from build123d import *

# Parameters (mm, degrees)
F0_R     = 1.905
F1_DEPTH = 2.032
F2_DEPTH = 2.54
F3_R     = 1.016


with BuildPart() as f1:
    # F0 (on Top) → F1 (new body)
    with BuildSketch(Plane.XY):
        with BuildLine():
            Line((6.35, 4.5080527947), (6.35, 7.0710607408))
            ThreePointArc((6.35, 7.0710607408), (3.4516559454, 8.1852117072), (0.3466541063, 8.1588637779))
            ThreePointArc((0.3466541063, 8.1588637779), (-4.4614598428, 5.2775997073), (-6.35, 1.93e-08))
            ThreePointArc((-6.35, 1.93e-08), (-4.4614598575, -5.2775996893), (0.3466540985, -8.1588637764))
            ThreePointArc((0.3466540985, -8.1588637764), (3.4516559415, -8.1852117079), (6.35, -7.0710607408))
            Line((6.35, -7.0710607408), (6.35, -4.5080527947))
            ThreePointArc((6.35, -4.5080527947), (-4.318, 0), (6.35, 4.5080527947))
        make_face()
        with BuildLine():
            Line((6.35, -4.5080527947), (6.35, 4.5080527947))
            ThreePointArc((6.35, 4.5080527947), (-4.318, 0), (6.35, -4.5080527947))
        make_face()
        with Locations((1.9685, 0)):
            Circle(F0_R, mode=Mode.SUBTRACT)
        with BuildLine():
            ThreePointArc((8.255, 0), (7.7591986625, 2.4470168062), (6.35, 4.5080527947))
            Line((6.35, 4.5080527947), (6.35, -4.5080527947))
            ThreePointArc((6.35, -4.5080527947), (7.7591986625, -2.4470168062), (8.255, 0))
        make_face()
        with BuildLine():
            ThreePointArc((10.287, 0), (9.2364071953, 4.0465994675), (6.35, 7.0710607408))
            Line((6.35, 7.0710607408), (6.35, 4.5080527947))
            ThreePointArc((6.35, 4.5080527947), (7.7591986625, 2.4470168062), (8.255, 0))
            ThreePointArc((8.255, 0), (7.7591986625, -2.4470168062), (6.35, -4.5080527947))
            Line((6.35, -4.5080527947), (6.35, -7.0710607408))
            ThreePointArc((6.35, -7.0710607408), (9.2364071953, -4.0465994675), (10.287, 0))
        make_face()
        with BuildLine():
            Line((-1.778, 9.9027430543), (-1.778, 12.7))
            Line((-1.778, 12.7), (-6.35, 12.7))
            Line((-6.35, 12.7), (-6.35, 1.93e-08))
            ThreePointArc((-6.35, 1.93e-08), (-4.4614598428, 5.2775997073), (0.3466541063, 8.1588637779))
            ThreePointArc((0.3466541063, 8.1588637779), (-1.1280365683, 8.528400484), (-1.778, 9.9027430543))
        make_face()
        with BuildLine():
            Line((6.35, 7.0710607408), (6.35, 12.7))
            Line((6.35, 12.7), (1.778, 12.7))
            Line((1.778, 12.7), (1.778, 9.9027430543))
            ThreePointArc((1.778, 9.9027430543), (1.3743425703, 8.774706486), (0.3466541063, 8.1588637779))
            ThreePointArc((0.3466541063, 8.1588637779), (3.4516559454, 8.1852117072), (6.35, 7.0710607408))
        make_face()
        with BuildLine():
            Line((6.35, -12.7), (6.35, -7.0710607408))
            ThreePointArc((6.35, -7.0710607408), (3.4516559415, -8.1852117079), (0.3466540985, -8.1588637764))
            ThreePointArc((0.3466540985, -8.1588637764), (1.3743425678, -8.7747064829), (1.778, -9.9027430543))
            Line((1.778, -9.9027430543), (1.778, -12.7))
            Line((1.778, -12.7), (6.35, -12.7))
        make_face()
        with BuildLine():
            ThreePointArc((0.3466540985, -8.1588637764), (-4.4614598575, -5.2775996893), (-6.35, 1.93e-08))
            Line((-6.35, 1.93e-08), (-6.35, -12.7))
            Line((-6.35, -12.7), (-1.778, -12.7))
            Line((-1.778, -12.7), (-1.778, -9.9027430543))
            ThreePointArc((-1.778, -9.9027430543), (-1.1280365714, -8.5284004866), (0.3466540985, -8.1588637764))
        make_face()
    extrude(amount=-F1_DEPTH)

    # F0 (on Top) → F2 (join)
    with BuildSketch(Plane.XY):
        with BuildLine():
            Line((6.35, 4.5080527947), (6.35, 7.0710607408))
            ThreePointArc((6.35, 7.0710607408), (3.4516559454, 8.1852117072), (0.3466541063, 8.1588637779))
            ThreePointArc((0.3466541063, 8.1588637779), (-4.4614598428, 5.2775997073), (-6.35, 1.93e-08))
            ThreePointArc((-6.35, 1.93e-08), (-4.4614598575, -5.2775996893), (0.3466540985, -8.1588637764))
            ThreePointArc((0.3466540985, -8.1588637764), (3.4516559415, -8.1852117079), (6.35, -7.0710607408))
            Line((6.35, -7.0710607408), (6.35, -4.5080527947))
            ThreePointArc((6.35, -4.5080527947), (-4.318, 0), (6.35, 4.5080527947))
        make_face()
        with BuildLine():
            ThreePointArc((10.287, 0), (9.2364071953, 4.0465994675), (6.35, 7.0710607408))
            Line((6.35, 7.0710607408), (6.35, 4.5080527947))
            ThreePointArc((6.35, 4.5080527947), (7.7591986625, 2.4470168062), (8.255, 0))
            ThreePointArc((8.255, 0), (7.7591986625, -2.4470168062), (6.35, -4.5080527947))
            Line((6.35, -4.5080527947), (6.35, -7.0710607408))
            ThreePointArc((6.35, -7.0710607408), (9.2364071953, -4.0465994675), (10.287, 0))
        make_face()
        with BuildLine():
            Line((6.35, 7.0710607408), (6.35, 12.7))
            Line((6.35, 12.7), (1.778, 12.7))
            Line((1.778, 12.7), (1.778, 9.9027430543))
            ThreePointArc((1.778, 9.9027430543), (1.3743425703, 8.774706486), (0.3466541063, 8.1588637779))
            ThreePointArc((0.3466541063, 8.1588637779), (3.4516559454, 8.1852117072), (6.35, 7.0710607408))
        make_face()
        with BuildLine():
            Line((-1.778, 9.9027430543), (-1.778, 12.7))
            Line((-1.778, 12.7), (-6.35, 12.7))
            Line((-6.35, 12.7), (-6.35, 1.93e-08))
            ThreePointArc((-6.35, 1.93e-08), (-4.4614598428, 5.2775997073), (0.3466541063, 8.1588637779))
            ThreePointArc((0.3466541063, 8.1588637779), (-1.1280365683, 8.528400484), (-1.778, 9.9027430543))
        make_face()
        with BuildLine():
            Line((6.35, -12.7), (6.35, -7.0710607408))
            ThreePointArc((6.35, -7.0710607408), (3.4516559415, -8.1852117079), (0.3466540985, -8.1588637764))
            ThreePointArc((0.3466540985, -8.1588637764), (1.3743425678, -8.7747064829), (1.778, -9.9027430543))
            Line((1.778, -9.9027430543), (1.778, -12.7))
            Line((1.778, -12.7), (6.35, -12.7))
        make_face()
        with BuildLine():
            ThreePointArc((0.3466540985, -8.1588637764), (-4.4614598575, -5.2775996893), (-6.35, 1.93e-08))
            Line((-6.35, 1.93e-08), (-6.35, -12.7))
            Line((-6.35, -12.7), (-1.778, -12.7))
            Line((-1.778, -12.7), (-1.778, -9.9027430543))
            ThreePointArc((-1.778, -9.9027430543), (-1.1280365714, -8.5284004866), (0.3466540985, -8.1588637764))
        make_face()
    extrude(amount=F2_DEPTH)

    # F3
    f3_edges = [f1.edges().sort_by_distance(p)[0] for p in [
        (-2.413, -4.508053, 2.54),
    ]]
    fillet(f3_edges, radius=F3_R)


solid = f1.part
The listing builds one solid part. Answer for the finished solid, in the listing's coordinates (mm). Coordinates: 2 decimals unless noted, no trailing zeros. Loops run counter-clockwise (first coordinate to the right, second up) from the corner with the lowest first, then second, coordinate; pieces in that order, holes last. Notation, with made-up numbers: (61, 36) -> (82, 36) arc R13 ccw to (82, 53) -> close; hole circle Ø4 at (83, -29). An arc over 180 degrees is marked (long way). Write item = value, one per line. Start each with the question number.
1) Given pin 1 Ø2 at (y, z) = (8.5, 1) entering from +X; pin 2 Ø2 at (y, z) = (-8.5, -1) entering from +X; pin 3 Ø2.5 at (x, y) = (1.97, 0) entering from +Z, each flat-ended and moving along its own axis, determine where each tip first touches the part or whether it passes through.
2) The mould has two halves that part along X. Classify faces 1 (the face through (0, -1, 0)), 2 (the face through (-2, 0, -2.032)), 3 (the face through (0.457, -1.159, -1.002)): released by +X, released by -X, zero draft, split by the parting line, or undercut.
3) A cutting plane is placed at B-B (y = 9). Give the vertices of the cut face in (x, z).
4) Straight lines are drawn through the part: line 1 (X direction, y = -10, z = -1.6); line 2 (X direction, y = 7.75, z = 0.45); line 3 (X direction, y = 0, z = 1) (3 decimals). For each, find the intervals that lie inside material, in ascending order. Write a range as from..to.
Responses:
q1.pin_1 = 6.35
q1.pin_2 = 6.35
q1.pin_3 = through
q2.face_1 = undercut
q2.face_2 = zero draft
q2.face_3 = undercut
q3.outline = (-6.35, -2.03) -> (-1.53, -2.03) -> (-1.53, 2.54) -> (-6.35, 2.54) -> close; (1.53, -2.03) -> (6.35, -2.03) -> (6.35, 2.54) -> (1.53, 2.54) -> close
q4.line_1 = -6.35..-1.78, 1.78..6.35
q4.line_2 = -6.35..6.35
q4.line_3 = -6.35..-4.318, 8.255..10.287
